from build123d import *

# Parameters (mm, degrees)
EXTRUDE_1_DEPTH     = 14
SKETCH_2_R          = 25
EXTRUDE_2_DEPTH     = 30
SKETCH_3_R          = 12.5
CUT_EXTRUDE_1_DEPTH = 78.638957463
SKETCH_4_W          = 15.8
SKETCH_4_H          = 8
CUT_EXTRUDE_2_DEPTH = 78.638957463
SKETCH_5_R          = 2.5
CUT_EXTRUDE_3_DEPTH = 12.6


with BuildPart() as part:
    # 草图1 → 凸台-拉伸1 (new body)
    with BuildSketch(Plane.XY):
        Polygon((33, 0), (32.877, 2.92), (32.509, 5.918), (31.905, 8.957), (31.082, 12.024), (30.05, 15.108), (28.805, 18.217), (27.368, 21.287), (25.721, 24.347), (23.877, 27.39), (21.833, 30.286), (19.566, 33.114), (17.058, 35.81), (14.33, 38.353), (11.355, 40.699), (8.143, 42.787), (4.705, 44.597), (1.07, 46.077), (-2.738, 47.178), (-6.695, 47.891), (-10.736, 48.154), (-14.831, 47.972), (-18.921, 47.32), (-22.957, 46.182), (-26.882, 44.596), (-30.655, 42.555), (-34.232, 40.082), (-37.587, 37.188), (-40.651, 33.948), (-43.421, 30.382), (-45.899, 26.5), (-48.034, 22.4), (-49.804, 18.127), (-51.194, 13.717), (-52.195, 9.203), (-52.798, 4.619), (-53, 0), (-52.792, -4.538), (-52.138, -8.965), (-51.069, -13.013), (-49.531, -16.93), (-47.557, -20.575), (-45.185, -23.874), (-42.441, -26.865), (-39.386, -29.472), (-36.063, -31.683), (-32.551, -33.456), (-28.863, -34.852), (-25.036, -35.873), (-21.187, -36.513), (-17.358, -36.81), (-13.57, -36.793), (-9.807, -36.517), (-6.123, -36.017), (-2.511, -35.329), (1.018, -34.495), (4.452, -33.532), (7.819, -32.438), (10.907, -31.265), (13.89, -29.95), (16.5, -28.579), (18.928, -27.032), (21.212, -25.279), (23.335, -23.335), (25.279, -21.212), (27.032, -18.928), (28.579, -16.5), (29.908, -13.946), (31.01, -11.287), (31.876, -8.541), (32.499, -5.73), (32.874, -2.876), align=None)
    extrude(amount=EXTRUDE_1_DEPTH)

    # 草图2 → 凸台-拉伸2 (add)
    with BuildSketch(Plane.XY):
        Circle(SKETCH_2_R)
    extrude(amount=EXTRUDE_2_DEPTH)

    # 草图3 → 切除-拉伸1 (cut, through all)
    with BuildSketch(Plane.XY):
        Circle(SKETCH_3_R)
    extrude(amount=CUT_EXTRUDE_1_DEPTH, mode=Mode.SUBTRACT)

    # 草图4 → 切除-拉伸2 (cut, through all)
    with BuildSketch(Plane.XY):
        with Locations((7.9, 0)):
            Rectangle(SKETCH_4_W, SKETCH_4_H)
    extrude(amount=CUT_EXTRUDE_2_DEPTH, mode=Mode.SUBTRACT)

    # 草图5 → 切除-拉伸3 (cut)
    with BuildSketch(Plane(origin=(25, 0, 0), x_dir=(0, 0, -1), z_dir=(1, 0, 0))):
        with Locations(Location((-22, 0, 0), (0, 0, 180))):
            Circle(SKETCH_5_R)
    extrude(amount=-CUT_EXTRUDE_3_DEPTH, mode=Mode.SUBTRACT)


solid = part.part
The model under review builds one solid part; all positions refer to its coordinate system, in mm. Round coordinates to 2 decimals unless told otherwise and drop trailing zeros. Write each loop counter-clockwise with the first axis right and the second up, starting at its lowest first coordinate (ties: lowest second). Pieces come first, ordered by that corner, then holes. Notation, with made-up numbers: (44.5, -25.5) - (84.5, -25.5) arc R35 cw to (84.5, 7.5) - close; hole circle Ø4 at (77.25, -17.75). An arc over 180 degrees is marked (long way). One line per item, written item: value. Start each with the question number.
1. Consider section A-A on x = 0. Write out the cut boundary in (y, z).
2. Clearance check with flat-ended pins moving along their axes: P1, Ø3, axis at x = 13.5, z = 16.5, coming from the -Y side; P2, Ø4, axis at x = -27, y = 30.5, coming from the -Z side; P3, Ø1.5, axis at x = 13.5, y = -27.5, coming from the +Z side; P4, Ø4.5, axis at x = 14.5, z = 7.5, coming from the +Y side. State where each tip first meets the part, or that it passes through.
3. The part is to be moulded in two halves that separate along Y. For faces 1 (the face through (20.5, -0.1, 19.5)), 2 (the face through (15.8, 0, 15)), 3 (the face through (22.87, 28.82, 6.9)), 4 (the face through (-48.558, -18.727, 6.902)), say which applies: released by +Y, released by -Y, zero draft, split by the parting line, or undercut.
4. Consider section B-B on z = 28.5. Write out the cut boundary in (x, y).
5. To check wall thickness, follow L1, parallel to X at y = 0, z = 10.75; L2, parallel to Z at x = -34.5, y = 14; L3, parallel to Y at x = 0, z = 19. State the ranges of each line that lie inside material, in increasing order. Write a range as from..to.
6. Consider section C-C on z = 22.5. Write out the cut boundary in (x, y), and give its area (3 significant figures).
Checks:
1. outline: (-34.74, 0) - (-12.5, 0) - (-12.5, 30) - (-25, 30) - (-25, 14) - (-34.74, 14) - close; (12.5, 0) - (46.39, 0) - (46.39, 14) - (25, 14) - (25, 30) - (12.5, 30) - close
2. P1: stops at y = -21.93
2. P2: stops at z = 0
2. P3: stops at z = 14
2. P4: stops at y = 39.99
3. face 1: undercut
3. face 2: undercut
3. face 3: released by +Y
3. face 4: released by -Y
4. outline: circle Ø50 at (0, 0); hole (11.84, -4) - (15.8, -4) - (15.8, 4) - (11.84, 4) arc R12.5 ccw (long way) to start
5. L1: x = -53..-12.5, 15.8..33
5. L2: z = 0..14
5. L3: y = -25..-12.5, 12.5..25
6. outline: (11.84, -4) arc R12.5 cw (long way) to (11.84, 4) - (15.8, 4) - (15.8, 2.45) - (24.88, 2.45) arc R25 ccw (long way) to (24.88, -2.45) - (15.8, -2.45) - (15.8, -4) - close
6. area: 1,400 mm^2
